For this review, take the finished solid that the model builds, in its own axes (mm). A direction names the side the tool comes from. Give positions to 0.01 mm unless a question says otherwise; leave off trailing zeros. Order: outer loops, then holes, each group sorted by start corner. A loop starts at its lowest first (then second) coordinate and runs counter-clockwise, first axis right, second up. Notation, with made-up numbers: (86.25, 69) -> (125.25, 69) arc R22 ccw to (125.25, 102) -> close; hole circle Ø2 at (50.25, 88.5). An arc over 180 degrees is marked (long way). One line per item, written item: value. Start each with the question number.
from build123d import *

# Parameters (mm, degrees)
ESQUISSE1_W        = 12.2
ESQUISSE1_H        = 15.8
BOSS_EXTRU_1_DEPTH = 3


with BuildPart() as part:
    # Esquisse1 → Boss.-Extru.1 (new body)
    with BuildSketch(Plane(origin=(0, 0, 0), x_dir=(1, 0, 0), z_dir=(0, 1, 0))):
        with BuildLine():
            Line((-9.5, 43), (-5, 43))
            Line((-5, 43), (-5, 46))
            Line((-5, 46), (5, 46))
            Line((5, 46), (5, 43))
            Line((5, 43), (9.5, 43))
            Line((9.5, 43), (9.5, 3))
            ThreePointArc((9.5, 3), (8.621320344, 0.878679656), (6.5, 0))
            Line((6.5, 0), (-6.5, 0))
            ThreePointArc((-6.5, 0), (-8.621320344, 0.878679656), (-9.5, 3))
            Line((-9.5, 3), (-9.5, 43))
        make_face()
        with Locations((0, 25.9)):
            Rectangle(ESQUISSE1_W, ESQUISSE1_H, mode=Mode.SUBTRACT)
    extrude(amount=BOSS_EXTRU_1_DEPTH)


solid = part.part
Q1. Take a section at D-D (x = 7.5). State the section outline as (y, z) points.
Q2. Take a section at A-A (y = 1.4). State the section outline as (x, z) points, and give its area (3 significant figures).
Q3. Take a section at C-C (z = -29.5). State the section outline as (x, y) points, and give its area (3 significant figures).
Q4. For pin 1 Ø1 at (x, y) = (-2.5, 1.5) entering from +Z; pin 2 Ø0.9 at (x, y) = (7.5, 1) entering from -Z, all flat-tipped, find the tip position at first contact; note any pin that passes through.
Q5. For faces 4 (the flat face through (-6.1, 1, -26)), 5 (the flat face through (5, 1, -45)), 6 (the cylindrical face through (8.64, 1.48, -0.9)), list the 3-axis set-ups (+Z, -Z, +X, -X, +Y, -Y) from which the entire face can be reached by the end or side of a thin tool; tool diameter is ignored.
Q6. For line 1 along Z through (x, y) = (3.25, 0.95); line 2 along X through (y, z) = (2.6, -26); line 3 along Z through (x, y) = (-6.5, 2.5), list the stretches that pass through material, from the lowest coordinate up.
Q7. Mouldability with a two-part tool opening along Z and no side actions: class faces 1 (the flat face through (-5, 1, -44)), 2 (the flat face through (-7, 1, -43)), 3 (the flat face through (0, 1, -18)) as pulls with the +Z half, pulls with the -Z half, needs draft (parallel to the pull), parting line crosses it, or undercut.
Q8. Take a section at B-B (x = 0). State the section outline as (y, z) points.
Answers below:
1. outline: (0, -43) -> (3, -43) -> (3, -0.17) -> (0, -0.17) -> close
2. outline: (-9.5, -43) -> (-5, -43) -> (-5, -46) -> (5, -46) -> (5, -43) -> (9.5, -43) -> (9.5, -3) arc R3 ccw to (6.5, 0) -> (-6.5, 0) arc R3 ccw to (-9.5, -3) -> close; hole (-6.1, -33.8) -> (6.1, -33.8) -> (6.1, -18) -> (-6.1, -18) -> close
2. area: 650 mm²
3. outline: (-9.5, 0) -> (-6.1, 0) -> (-6.1, 3) -> (-9.5, 3) -> close; (6.1, 0) -> (9.5, 0) -> (9.5, 3) -> (6.1, 3) -> close
3. area: 20.4 mm²
4. pin 1: stops at z = 0
4. pin 2: stops at z = -43
5. face 4: +Y, -Y
5. face 5: -Z, +X, +Y, -Y
5. face 6: +Z, +X, +Y, -Y
6. line 1: z = -46 to -33.8, -18 to 0
6. line 2: x = -9.5 to -6.1, 6.1 to 9.5
6. line 3: z = -43 to 0
7. face 1: needs draft
7. face 2: pulls with the -Z half
7. face 3: undercut
8. outline: (0, -46) -> (3, -46) -> (3, -33.8) -> (0, -33.8) -> close; (0, -18) -> (3, -18) -> (3, 0) -> (0, 0) -> close
